Geometry check sheet. Reference: the model listing, model coordinates, mm. A direction names the side the tool comes from. Coordinates: 2 decimals unless noted, no trailing zeros. Order: outer loops, then holes, each group sorted by start corner. A loop starts at its lowest first (then second) coordinate and runs counter-clockwise, first axis right, second up. Notation, with made-up numbers: (28, 15.5) -> (56, 15.5) arc R16 cw to (56, 28.5) -> close; hole circle Ø3 at (71.5, 19.5). An arc over 180 degrees is marked (long way). Answer as CSV lines item,"result". Start each with the question number.
from build123d import *

# Parameters (mm, degrees)
EXTRUDE_1_DEPTH = 10


with BuildPart() as part:
    # 草图1 → 凸台-拉伸1 (new body)
    with BuildSketch(Plane.XY):
        with BuildLine():
            ThreePointArc((-12, 248), (-11.22497216, 243.757359313), (-9, 240.062746067))
            Line((-9, 240.062746067), (-9, 248))
            ThreePointArc((-9, 248), (0, 257), (9, 248))
            Line((9, 248), (9, 240.062746067))
            ThreePointArc((9, 240.062746067), (11.22497216, 243.757359313), (12, 248))
            ThreePointArc((12, 248), (0, 260), (-12, 248))
        make_face()
        with BuildLine():
            ThreePointArc((-12, 0), (-11.22497216, 4.242640687), (-9, 7.937253933))
            Line((-9, 7.937253933), (-9, 240.062746067))
            ThreePointArc((-9, 240.062746067), (-11.22497216, 243.757359313), (-12, 248))
            Line((-12, 248), (-12, 0))
        make_face()
        with BuildLine():
            Line((9, 240.062746067), (9, 7.937253933))
            ThreePointArc((9, 7.937253933), (11.22497216, 4.242640687), (12, 0))
            Line((12, 0), (12, 248))
            ThreePointArc((12, 248), (11.22497216, 243.757359313), (9, 240.062746067))
        make_face()
        with BuildLine():
            Line((9, 7.937253933), (9, 0))
            ThreePointArc((9, 0), (0, -9), (-9, 0))
            Line((-9, 0), (-9, 7.937253933))
            ThreePointArc((-9, 7.937253933), (-11.22497216, 4.242640687), (-12, 0))
            ThreePointArc((-12, 0), (0, -12), (12, 0))
            ThreePointArc((12, 0), (11.22497216, 4.242640687), (9, 7.937253933))
        make_face()
    extrude(amount=EXTRUDE_1_DEPTH)


solid = part.part
Q1. Sectioned sample at A-A, the plane x = 0. Record the cut outline in (y, z).
Q2. Thickness scan on L1, parallel to X at y = 119, z = 5.5; L2, parallel to Y at x = 0.5, z = 8.25; L3, parallel to Y at x = -6.5, z = 4. Record the ranges inside material, lowest first.
Q3. Sectioned sample at B-B, the plane y = 115. Record the cut outline in (x, z).
Q4. Go/stop test with flat-tipped pins: pin 1 Ø1.5 at (x, z) = (5, 2.5) entering from -Y; pin 2 Ø4 at (x, z) = (-9, 8) entering from +Y. Record where each tip stops, or that it passes through.
Q5. Release check for a two-part mould opening along X. For faces 3 (the flat face through (9, 126, 5)), 4 (the flat face through (11, 115, 0)), 5 (the flat face through (12, 122, 5)) record: released by +X, released by -X, zero draft, split by the parting line, or undercut.
Q6. Sectioned sample at C-C, the plane z = 3.75. Record the cut outline in (x, y).
Q7. Access from +Z, -Z, +X, -X, +Y, -Y to the whole of each face (thin tool, end or side, straight path). Record for faces 1 (the flat face through (11, 115, 10)), 2 (the cylindrical face through (0, 257, 5)).
Geometry results:
1,outline,"(-12, 0) -> (-9, 0) -> (-9, 10) -> (-12, 10) -> close; (257, 0) -> (260, 0) -> (260, 10) -> (257, 10) -> close"
2,L1,"x = -12 to -9, 9 to 12"
2,L2,"y = -11.99 to -8.99, 256.99 to 259.99"
2,L3,"y = -10.09 to -6.22, 254.22 to 258.09"
3,outline,"(-12, 0) -> (-9, 0) -> (-9, 10) -> (-12, 10) -> close; (9, 0) -> (12, 0) -> (12, 10) -> (9, 10) -> close"
4,pin 1,"stops at y = -11.22"
4,pin 2,"stops at y = 257.75"
5,face 3,"undercut"
5,face 4,"zero draft"
5,face 5,"released by +X"
6,outline,"(-12, 0) arc R12 ccw to (12, 0) -> (12, 248) arc R12 ccw to (-12, 248) -> close; hole (-9, 0) arc R9 ccw to (9, 0) -> (9, 248) arc R9 ccw to (-9, 248) -> close"
7,face 1,"+Z, +X, -X, +Y, -Y"
7,face 2,"+Z, -Z"
